```python
from build123d import *

# Parameters (mm, degrees)
SKETCH1_W           = 5.08
SKETCH1_H           = 6.35
SKETCH1_W_2         = 27.686
SKETCH1_H_2         = 28.575
SKETCH1_R           = 10.668
BOSS_EXTRUDE1_DEPTH = 5.08


with BuildPart() as part:
    # Sketch1 → Boss-Extrude1 (new body)
    with BuildSketch(Plane(origin=(0, 0, 0), x_dir=(1, 0, 0), z_dir=(0, 1, 0))):
        with Locations((-16.383, -11.1125)):
            Rectangle(SKETCH1_W, SKETCH1_H)
        with Locations((-16.383, 11.1125)):
            Rectangle(SKETCH1_W, SKETCH1_H)
        Rectangle(SKETCH1_W_2, SKETCH1_H_2)
        Circle(SKETCH1_R, mode=Mode.SUBTRACT)
        with Locations((16.383, 11.1125)):
            Rectangle(SKETCH1_W, SKETCH1_H)
        with Locations((16.383, -11.1125)):
            Rectangle(SKETCH1_W, SKETCH1_H)
    extrude(amount=BOSS_EXTRUDE1_DEPTH)


solid = part.part
```
For this review, take the finished solid that the model builds, in its own axes (mm). A direction names the side the tool comes from. Round coordinates to 2 decimals unless told otherwise and drop trailing zeros. Write each loop counter-clockwise with the first axis right and the second up, starting at its lowest first coordinate (ties: lowest second). Pieces come first, ordered by that corner, then holes. Notation, with made-up numbers: (39, 56) - (67, 56) arc R22 cw to (67, 75) - close; hole circle Ø10 at (78.5, 48). An arc over 180 degrees is marked (long way). Put each result on its own line as item: value.
Q1. Insertion check: pin 1 Ø2 at (y, z) = (1, -2.5) entering from +X. The pin has a flat end and moves straight along its axis. Give the tip position at first contact, or say it passes through.
Solved:
pin 1: stops at x = 13.84
Q2. Mouldability with a two-part tool opening along Z and no side actions: class faces 4 (the face through (-16, 3, -7.938)), 5 (the face through (-9, 5.08, -7)), 6 (the face through (0, 3, 14.288)) as released by +Z, released by -Z, zero draft, split by the parting line, or undercut.
Solved:
face 4: undercut
face 5: zero draft
face 6: released by +Z
Q3. Machinability: for faces 1 (the face through (-18.923, 3, 11)), 2 (the face through (13.843, 3, 0)), 3 (the face through (-13.843, 3, 0)), which of the approach directions +Z, -Z, +X, -X, +Y, -Y give a long, thin tool a straight path to every point of the face, cutting with its end or side? Answer none if there is none.
Solved:
face 1: +Z, -Z, -X, +Y, -Y
face 2: +X, +Y, -Y
face 3: -X, +Y, -Y
Q4. Wall thickness on probe 1 along Z at (x, y) = (16, 2.3); probe 2 along Z at (x, y) = (0, 3.35); probe 3 along X at (y, z) = (3.15, 0): over which ranges is each line inside the solid? List them lowest first.
Solved:
probe 1: z = -14.29 to -7.94, 7.94 to 14.29
probe 2: z = -14.29 to -10.67, 10.67 to 14.29
probe 3: x = -13.84 to -10.67, 10.67 to 13.84
Q5. We need section C-C (y = 4.5). Give the boundary of the cut face in (x, z), and give its area (3 significant figures).
Solved:
outline: (-18.92, -14.29) - (18.92, -14.29) - (18.92, -7.94) - (13.84, -7.94) - (13.84, 7.94) - (18.92, 7.94) - (18.92, 14.29) - (-18.92, 14.29) - (-18.92, 7.94) - (-13.84, 7.94) - (-13.84, -7.94) - (-18.92, -7.94) - close; hole circle Ø21.34 at (0, 0)
area: 563 mm2
Q6. We need section B-B (x = 16). Give the boundary of the cut face in (y, z), and give its area (3 significant figures).
Solved:
outline: (0, -14.29) - (5.08, -14.29) - (5.08, -7.94) - (0, -7.94) - close; (0, 7.94) - (5.08, 7.94) - (5.08, 14.29) - (0, 14.29) - close
area: 64.5 mm2
Q7. We need section A-A (z = 0). Give the boundary of the cut face in (x, y).
Solved:
outline: (-13.84, 0) - (-10.67, 0) - (-10.67, 5.08) - (-13.84, 5.08) - close; (10.67, 0) - (13.84, 0) - (13.84, 5.08) - (10.67, 5.08) - close
